Check sheet for the drawn part. Datum: minimum x, y, z corner. Units: mm. A direction names the side the tool comes from. Give positions to 0.01 mm unless a question says otherwise; leave off trailing zeros. Write each loop counter-clockwise with the first axis right and the second up, starting at its lowest first coordinate (ties: lowest second). Pieces come first, ordered by that corner, then holes. Notation, with made-up numbers: (61.25, -10.5) - (98.25, -10.5) arc R28 ccw to (98.25, 21.5) - close; hole circle Ø2 at (61.5, -38.75). An arc over 180 degrees is marked (long way). Answer as a JSON object with one key per item and string values. Group by question number.
Item 1: Go/stop test with flat-tipped pins: pin 1 (3 mm diameter, centred on y = 17, z = 7.5, fed in from +X); pin 2 (5 mm diameter, centred on x = 6, z = 13, fed in from -Y). Record where each tip stops, or that it passes through.
Item 2: Sectioned sample at B-B, the plane z = 14.5. Record the boundary of the cut face in (x, y).
Item 3: Scan lines: line 1 along Z through (x, y) = (6.5, 26.6); line 2 along Y through (x, z) = (1.5, 6); line 3 along Y through (x, z) = (3, 6). Record each from-to range of solid material in increasing order. Write a range as [from, to].
Item 4: Sectioned sample at D-D, the plane y = 23.5. Record the boundary of the cut face in (x, z), and give its area (3 significant figures).
Item 5: Sectioned sample at A-A, the plane x = 6.5. Record the boundary of the cut face in (y, z), and give its area (3 significant figures).
Item 6: Tool access check on the marked faces 1 and 2. Record the directions out of +Z, -Z, +X, -X, +Y, -Y that give a thin tool (end or side, any length) a straight path to the whole face; none if there is none.
Item 7: Sectioned sample at C-C, the plane z = 6.5. Record the boundary of the cut face in (x, y).
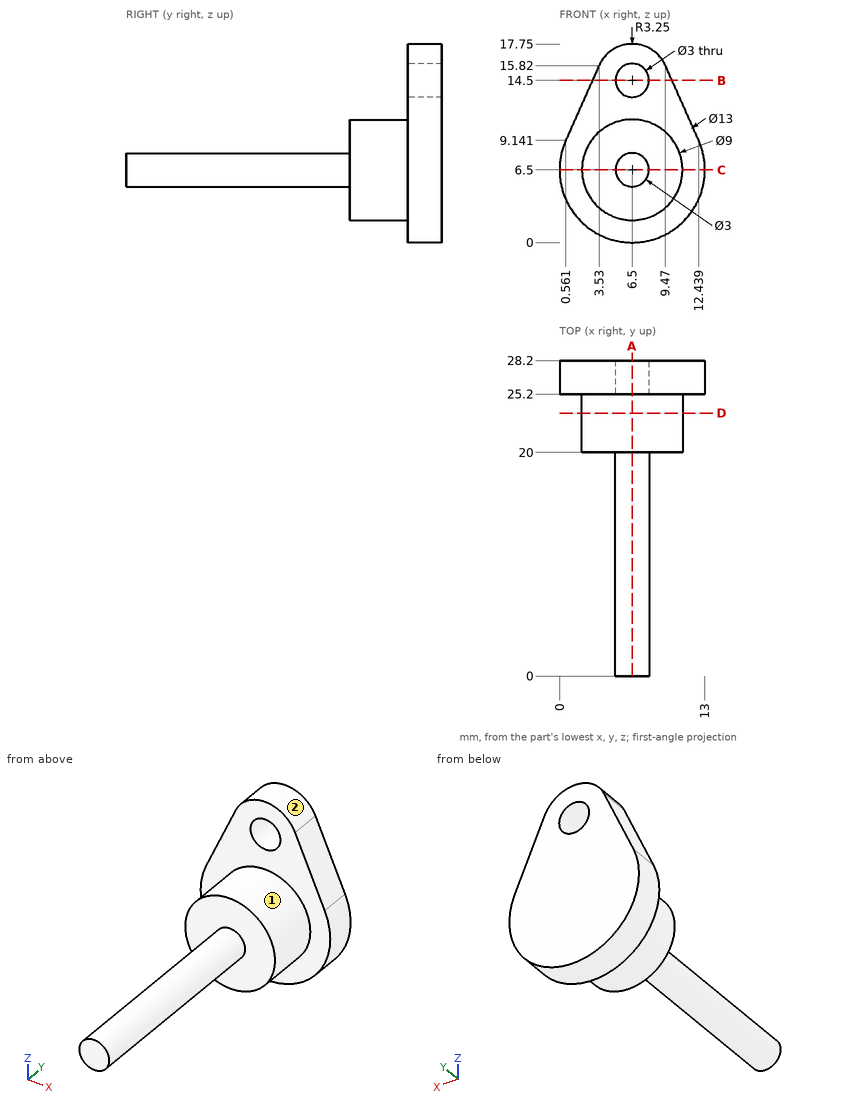
Geometry check:
{
 "1": {"pin 1": "x = 8", "pin 2": "y = 20"},
 "2": {"outline": "(2.94, 25.2) - (5, 25.2) - (5, 28.2) - (2.94, 28.2) - close; (8, 25.2) - (10.06, 25.2) - (10.06, 28.2) - (8, 28.2) - close"},
 "3": {"line 1": "[0, 13], [16, 17.75]", "line 2": "[25.2, 28.2]", "line 3": "[20, 28.2]"},
 "4": {"outline": "circle Ø9 at (6.5, 6.5)", "area": "63.6 mm^2"},
 "5": {"outline": "(0, 5) - (20, 5) - (20, 2) - (25.2, 2) - (25.2, 0) - (28.2, 0) - (28.2, 13) - (25.2, 13) - (25.2, 11) - (20, 11) - (20, 8) - (0, 8) - close; (25.2, 16) - (28.2, 16) - (28.2, 17.75) - (25.2, 17.75) - close", "area": "151 mm^2"},
 "6": {"face 1": "-Y", "face 2": "+Z, +Y, -Y"},
 "7": {"outline": "(0, 25.2) - (2, 25.2) - (2, 20) - (5, 20) - (5, 0) - (8, 0) - (8, 20) - (11, 20) - (11, 25.2) - (13, 25.2) - (13, 28.2) - (0, 28.2) - close"}
}
